Can you work these out from the model? Positions are in its coordinate system, mm. A direction names the side the tool comes from. Round coordinates to 2 decimals unless told otherwise and drop trailing zeros. Write each loop counter-clockwise with the first axis right and the second up, starting at its lowest first coordinate (ties: lowest second). Pieces come first, ordered by that corner, then holes. Notation, with made-up numbers: (67, 3.25) -> (88, 3.25) arc R19 cw to (88, 25.25) -> close; hole circle Ø6 at (-7, -11.5). An arc over 180 degrees is marked (long way). Write item = value, one per line. Start each with the question number.
1) If I drill on line 1 (X direction, y = -9, z = 1.8); line 2 (X direction, y = -47, z = 3); line 3 (X direction, y = -52, z = 1.05), over which ranges is the centre line in solid material (lowest first)?
2) I'm going to push flat-ended pins straight in: pin 1 (1.6 mm diameter, centred on x = 54, z = 2.5, fed in from -Y); pin 2 (1 mm diameter, centred on y = -30.5, z = 1.5, fed in from +X); pin 3 (1.6 mm diameter, centred on y = -16.5, z = 1, fed in from -X). Where does each tip first touch, or does it pass through?
3) For faces 1 (the face through (-50.8, -10, 2)), 2 (the face through (57, 24.587, 2)), 3 (the face through (-29.58, -50.03, 1.57)), which set-ups out of +Z, -Z, +X, -X, +Y, -Y let a thin tool reach every point of the face, with its end or its side?
4) Imagine slicing it at A-A, the plane y = -59. Please give me the cut outline in (x, z) (3 decimals).
5) Imagine slicing it at C-C, the plane y = 0. Please give me the cut outline in (x, z) (3 decimals).
6) Imagine slicing it at D-D, the plane x = 48. Please give me the cut outline in (y, z) (3 decimals).
7) Thinking about a two-plate mould opening in Y: for faces 4 (the face through (-1, 4, 3.175)), 5 (the face through (-57, -44.983, 2)), 6 (the face through (-0.038, -33.128, 1.61)), which applies, +Y half, -Y half, draft (parallel to the pull), parting line (faces both ways), or undercut?
8) Imagine slicing it at B-B, the plane z = 1.55. Please give me the cut outline in (x, y).
from build123d import *

# Parameters (mm, degrees)
F0_W     = 12.7
F0_H     = 22.5932470911
F1_DEPTH = 3.175
F2_R     = 5.08


# Not quite as in the source:
# - two fillets or chamfers of one size are made in one step
# - a feature names something its author has since deleted; it is built from what else it names


with BuildPart() as f1:
    # F0 (on Top) → F1 (new body)
    with BuildSketch(Plane.XY):
        Polygon((-50.8, 47.1803817213), (-50.8, 24.5871346301), (-50.8, -32.2834653699), (-50.8, -44.9834653699), (-63.5, -44.9834653699), (-63.5, -70.3834653699), (0, -32.2834653699), (63.5, -70.3834653699), (63.5, -44.9834653699), (50.8, -44.9834653699), (50.8, -32.2834653699), (50.8, 24.5871346301), (50.8, 47.1803817213), (0, 47.1803817213), align=None)
        with Locations((-57.15, 35.8837581757)):
            Rectangle(F0_W, F0_H)
        with Locations((57.15, 35.8837581757)):
            Rectangle(F0_W, F0_H)
    extrude(amount=F1_DEPTH)

    # F2
    f2_edges = [f1.edges().sort_by_distance(p)[0] for p in [
        (-63.5, -70.383465, 1.5875),
        (0, -32.283465, 1.5875),
        (63.5, -70.383465, 1.5875),
    ]]
    fillet(f2_edges, radius=F2_R)


solid = f1.part
Reported:
q1.line_1 = -50.8 to 50.8
q1.line_2 = -63.5 to -24.53, 24.53 to 63.5
q1.line_3 = -63.5 to -32.86, 32.86 to 63.5
q2.pin_1 = -65.16
q2.pin_2 = 50.8
q2.pin_3 = -50.8
q3.face_1 = +Z, -Z, -X
q3.face_2 = +Z, -Z, +X
q3.face_3 = +Z, -Z, -Y
q4.outline = (-63.5, 0) -> (-44.528, 0) -> (-44.528, 3.175) -> (-63.5, 3.175) -> close; (44.528, 0) -> (63.5, 0) -> (63.5, 3.175) -> (44.528, 3.175) -> close
q5.outline = (-50.8, 0) -> (50.8, 0) -> (50.8, 3.175) -> (-50.8, 3.175) -> close
q6.outline = (-61.083, 0) -> (47.18, 0) -> (47.18, 3.175) -> (-61.083, 3.175) -> close
q7.face_4 = draft
q7.face_5 = undercut
q7.face_6 = -Y half
q8.outline = (-63.5, -61.41) arc R5.08 ccw to (-55.81, -65.77) -> (-2.61, -33.85) arc R5.08 cw to (2.61, -33.85) -> (55.81, -65.77) arc R5.08 ccw to (63.5, -61.41) -> (63.5, -44.98) -> (50.8, -44.98) -> (50.8, 24.59) -> (63.5, 24.59) -> (63.5, 47.18) -> (-63.5, 47.18) -> (-63.5, 24.59) -> (-50.8, 24.59) -> (-50.8, -44.98) -> (-63.5, -44.98) -> close
